```python
from build123d import *
from build123d.topology import SkipClean

# Parameters (mm, degrees)
SKETCH1_W             = 8
SKETCH1_H             = 19
SKETCH1_R             = 1.5
BOSS_EXTRUDE1_DEPTH   = 2
BOSS_EXTRUDE1_2_DEPTH = 2
SKETCH3_W             = 8
SKETCH3_H             = 2
BOSS_EXTRUDE3_DEPTH   = 4.5
SKETCH4_W             = 9
SKETCH4_H             = 18.077551635
BOSS_EXTRUDE4_DEPTH   = 9
BOSS_EXTRUDE5_DEPTH   = 18.077552
SKETCH6_R             = 1.5
CUT_EXTRUDE1_DEPTH    = 57.189837927
SKETCH1_3_R           = 1.5
CUT_EXTRUDE2_DEPTH    = 55.158745093
SKETCH1_4_R           = 1.5
CUT_EXTRUDE3_DEPTH    = 55.158745093
SKETCH12_W            = 42
SKETCH12_H            = 2
CUT_EXTRUDE5_DEPTH    = 1.5
BOSS_EXTRUDE6_START   = 2
SKETCH14_R            = 1.5
BOSS_EXTRUDE6_DEPTH   = 2
FILLET1_R             = 1


with BuildPart() as part:
    # Sketch1 → Boss-Extrude1 (new body)
    with BuildSketch(Plane(origin=(0, 0, 0), x_dir=(1, 0, 0), z_dir=(0, 1, 0))):
        with Locations((-4.5, 10)):
            Rectangle(SKETCH1_W, SKETCH1_H)
        with Locations(Location((-4.5, 15, 0), (0, 0, 270))):
            Circle(SKETCH1_R, mode=Mode.SUBTRACT)
        with Locations(Location((-4.5, 5, 0), (0, 0, 270))):
            Circle(SKETCH1_R, mode=Mode.SUBTRACT)
    extrude(amount=BOSS_EXTRUDE1_DEPTH)



with BuildPart() as body_2:
    # Sketch1 → Boss-Extrude1 2 (new body)
    with BuildSketch(Plane(origin=(0, 0, 0), x_dir=(1, 0, 0), z_dir=(0, 1, 0))):
        with Locations((45.5, 10)):
            Rectangle(SKETCH1_W, SKETCH1_H)
    extrude(amount=BOSS_EXTRUDE1_2_DEPTH)


with BuildPart() as part_1:
    add(part.part)

    add(body_2.part)  # Boss-Extrude3 merges body 2
    # Sketch3 → Boss-Extrude3 (add)
    with BuildSketch(Plane.XY.offset(-0.5)):
        Polygon((-0.5, 2), (-0.5, 0), (49.5, 0), (49.5, 7.944947695), (-8.5, 7.944947695), (-8.5, 2), align=None)
        Polygon((-0.5, 0), (-8.5, 0), (-8.5, -10.13260394), (49.5, -10.13260394), (49.5, 0), align=None)
        with Locations((-4.5, 1)):
            Rectangle(SKETCH3_W, SKETCH3_H)
    extrude(amount=BOSS_EXTRUDE3_DEPTH)

    # Sketch4 → Boss-Extrude4 (add)
    with BuildSketch(Plane.XY.offset(4)):
        with Locations((20, -1.093828123)):
            Rectangle(SKETCH4_W, SKETCH4_H)
    extrude(amount=BOSS_EXTRUDE4_DEPTH)

    # Sketch5 → Boss-Extrude5 (add, through all)
    with BuildSketch(Plane(origin=(0, 7.944947695, 0), x_dir=(1, 0, 0), z_dir=(0, 1, 0))):
        with BuildLine():
            Line((18.5, -13), (15.5, -13))
            ThreePointArc((15.5, -13), (20, -17.5), (24.5, -13))
            Line((24.5, -13), (21.5, -13))
            ThreePointArc((21.5, -13), (20, -14.5), (18.5, -13))
        make_face()
    extrude(amount=-BOSS_EXTRUDE5_DEPTH)

    # Sketch6 → Cut-Extrude1 (cut, through all)
    with SkipClean():  # the faces are left unmerged after this step: merging them gives an invalid solid
        with BuildSketch(Plane(origin=(0, 7.944947695, 0), x_dir=(1, 0, 0), z_dir=(0, 1, 0))):
            with Locations(Location((20, -13, 0), (0, 0, 270))):
                Circle(SKETCH6_R)
        extrude(amount=-CUT_EXTRUDE1_DEPTH, mode=Mode.SUBTRACT)

    # Sketch1<3> → Cut-Extrude2 (cut, through all)
    with SkipClean():  # the faces are left unmerged after this step: merging them gives an invalid solid
        with BuildSketch(Plane(origin=(0, 0, 0), x_dir=(1, 0, 0), z_dir=(0, 1, 0))):
            with Locations(Location((45.5, 15, 0), (0, 0, 90))):
                Circle(SKETCH1_3_R)
        extrude(amount=CUT_EXTRUDE2_DEPTH, mode=Mode.SUBTRACT)

    # Sketch1<4> → Cut-Extrude3 (cut, through all)
    with SkipClean():  # the faces are left unmerged after this step: merging them gives an invalid solid
        with BuildSketch(Plane(origin=(0, 0, 0), x_dir=(1, 0, 0), z_dir=(0, 1, 0))):
            with Locations(Location((45.5, 5, 0), (0, 0, 90))):
                Circle(SKETCH1_4_R)
        extrude(amount=CUT_EXTRUDE3_DEPTH, mode=Mode.SUBTRACT)

    # Sketch12 → Cut-Extrude5 (cut)
    with SkipClean():  # the faces are left unmerged after this step: merging them gives an invalid solid
        with BuildSketch(Plane(origin=(0, 0, -0.5), x_dir=(-1, 0, 0), z_dir=(0, 0, -1))):
            Polygon((-41.5, 2), (0.5, 2), (8.5, 2), (8.5, 7.944947695), (-49.5, 7.944947695), (-49.5, 2), align=None)
            with Locations((-20.5, 1)):
                Rectangle(SKETCH12_W, SKETCH12_H)
            Polygon((-41.5, 0), (-49.5, 0), (-49.5, -10.13260394), (8.5, -10.13260394), (8.5, 0), (0.5, 0), align=None)
        extrude(amount=-CUT_EXTRUDE5_DEPTH, mode=Mode.SUBTRACT)

    # Sketch14 → Boss-Extrude6 (add)
    with BuildSketch(Plane(origin=(0, 7.944947695, 0), x_dir=(1, 0, 0), z_dir=(0, 1, 0)).offset(BOSS_EXTRUDE6_START)):
        with BuildLine():
            Line((49.5, -1), (-8.5, -1))
            Line((-8.5, -1), (-8.5, -4))
            Line((-8.5, -4), (15.5, -4))
            Line((15.5, -4), (15.5, -13))
            ThreePointArc((15.5, -13), (20, -17.5), (24.5, -13))
            Line((24.5, -13), (24.5, -4))
            Line((24.5, -4), (49.5, -4))
            Line((49.5, -4), (49.5, -1))
        make_face()
        with Locations(Location((20, -13, 0), (0, 0, 270))):
            Circle(SKETCH14_R, mode=Mode.SUBTRACT)
    extrude(amount=-BOSS_EXTRUDE6_DEPTH)

    # Fillet1
    fillet1_edges = [part_1.edges().sort_by_distance(p)[0] for p in [
        (-0.5, 2, -9.25),
        (45.5, 2, 1),
        (49.5, 5.972473847, 1),
        (-8.5, 5.972473847, 1),
        (-4.5, 2, 1),
        (-0.5, 1, 1),
        (-8.5, -5.06630197, 1),
        (20.5, -10.13260394, 1),
        (49.5, -5.06630197, 1),
        (41.5, 1, 1),
        (20, 9.944947695, 17.5),
        (24.5, 9.944947695, 8.5),
        (37, 9.944947695, 4),
        (20.5, 9.944947695, 1),
        (-8.5, 9.944947695, 2.5),
        (-4.5, 2, -19.5),
        (3.5, 9.944947695, 4),
        (15.5, 9.944947695, 8.5),
        (-8.5, 2, -9.25),
        (-8.5, -0.093828123, 4),
        (-8.5, -10.13260394, 2.5),
        (3.5, -10.13260394, 4),
        (49.5, -0.093828123, 4),
        (49.5, 2, -9.25),
        (45.5, 2, -19.5),
        (41.5, 2, -9.25),
        (37, -10.13260394, 4),
        (15.5, -10.13260394, 8.5),
        (24.5, -0.093828123, 4),
        (24.5, -10.13260394, 8.5),
        (15.5, -0.093828123, 4),
        (20, -10.132604305, 17.5),
    ]]
    fillet(fillet1_edges, radius=FILLET1_R)


solid = part_1.part
```
Read the model definition and answer for the solid it produces. Units are mm, in the model's axes. A direction names the side the tool comes from. Round coordinates to 2 decimals unless told otherwise and drop trailing zeros. Write each loop counter-clockwise with the first axis right and the second up, starting at its lowest first coordinate (ties: lowest second). Pieces come first, ordered by that corner, then holes. Notation, with made-up numbers: (37, 61) -> (93, 61) arc R19 ccw to (93, 73) -> close; hole circle Ø5 at (47, 48.5). An arc over 180 degrees is marked (long way). Answer in a Markdown table with one row per item. Add a question column.
1) Consider line 1 (Z direction, x = 45.5, y = 0.7); line 2 (X direction, y = 0.75, z = -5); line 3 (Z direction, x = 20, y = 3.75). Determine where each line is inside the solid, lowest interval first.
2) Find section C-C, the plane y = -5. Determine the outline of the cut face in (x, z).
3) Given P1, Ø2.5, axis at x = 45.5, z = -5, coming from the -Y side; P2, Ø9, axis at x = 2, y = -3, coming from the +Z side; P3, Ø7, axis at x = 45.5, z = -7.5, coming from the -Y side; P4, Ø10, axis at x = 28, y = 2, coming from the +Z side, each flat-ended and moving along its own axis, determine where each tip first touches the part or whether it passes through.
4) Find section A-A, the plane x = 20. Determine the outline of the cut face in (y, z).
5) Find section B-B, the plane z = -10. Determine the outline of the cut face in (x, y), and give its area (3 significant figures).
6) Which of the six approach directions +Z, -Z, +X, -X, +Y, -Y give full straight-line access (tool end or side, diameter ignored) to faces 1 (the face through (-4, 2, -9)), 2 (the face through (3, 0, 4)), 3 (the face through (24.5, 0, 9))?
7) Find section D-D, the plane z = -15. Determine the outline of the cut face in (x, y).
Findings below:
| question | item | result |
|---|---|---|
| 1 | line 1 | -19.5 to -16.5, -13.5 to -6.5, -3.5 to 4 |
| 1 | line 2 | -8.5 to -6, -3 to -0.5, 41.5 to 44, 47 to 49.5 |
| 1 | line 3 | 1 to 11.5, 14.5 to 17.5 |
| 2 | outline | (-8.5, 2) arc R1 ccw to (-7.5, 1) -> (48.5, 1) arc R1 ccw to (49.5, 2) -> (49.5, 3) arc R1 ccw to (48.5, 4) -> (25.5, 4) arc R1 cw to (24.5, 5) -> (24.5, 13) arc R4.5 ccw to (15.5, 13) -> (15.5, 5) arc R1 cw to (14.5, 4) -> (-7.5, 4) arc R1 ccw to (-8.5, 3) -> close; hole circle Ø3 at (20, 13) |
| 3 | P1 | through |
| 3 | P2 | z = 4 |
| 3 | P3 | y = 0 |
| 3 | P4 | z = 16.35 |
| 4 | outline | (-10.13, 2) arc R1 ccw to (-9.13, 1) -> (8.94, 1) arc R1 ccw to (9.94, 2) -> (9.94, 11.5) -> (-10.13, 11.5) -> close; (-10.13, 14.5) -> (9.94, 14.5) -> (9.94, 16.5) arc R1 ccw to (8.94, 17.5) -> (-9.13, 17.5) arc R1 ccw to (-10.13, 16.5) -> close |
| 5 | outline | (-8.5, 0) -> (-0.5, 0) -> (-0.5, 1) arc R1 ccw to (-1.5, 2) -> (-7.5, 2) arc R1 ccw to (-8.5, 1) -> close; (41.5, 0) -> (49.5, 0) -> (49.5, 1) arc R1 ccw to (48.5, 2) -> (42.5, 2) arc R1 ccw to (41.5, 1) -> close |
| 5 | area | 31.1 mm² |
| 6 | face 1 | -Z, +X, -X, +Y |
| 6 | face 2 | +Z, -X, +Y, -Y |
| 6 | face 3 | +Z, +X, +Y, -Y |
| 7 | outline | (-8.5, 0) -> (-6, 0) -> (-6, 2) -> (-7.5, 2) arc R1 ccw to (-8.5, 1) -> close; (-3, 0) -> (-0.5, 0) -> (-0.5, 1) arc R1 ccw to (-1.5, 2) -> (-3, 2) -> close; (41.5, 0) -> (44, 0) -> (44, 2) -> (42.5, 2) arc R1 ccw to (41.5, 1) -> close; (47, 0) -> (49.5, 0) -> (49.5, 1) arc R1 ccw to (48.5, 2) -> (47, 2) -> close |
